Verification items for the finished model (mm, model axes). A direction names the side the tool comes from. Give positions to 0.01 mm unless a question says otherwise; leave off trailing zeros. Write each loop counter-clockwise with the first axis right and the second up, starting at its lowest first coordinate (ties: lowest second). Pieces come first, ordered by that corner, then holes. Notation, with made-up numbers: (4.5, 13.5) -> (9.5, 13.5) arc R19 cw to (9.5, 37.5) -> close; hole circle Ø5 at (36, 51.25). An arc over 180 degrees is marked (long way). Write item = value, one per line.
from build123d import *

# Parameters (mm, degrees)
PAD011_DEPTH                = 4.6
SKETCH016_W                 = 26.6
SKETCH016_H                 = 26.6
POCKET005_DEPTH             = 3.6
SKETCH018_R                 = 2.032
SKETCH018_R_2               = 0.832
PAD012_DEPTH                = 2
SKETCH018_MIRRORED013_2_R   = 2.032
SKETCH018_MIRRORED013_2_R_2 = 0.832
PAD012_MIRRORED013_2_DEPTH  = 2
SKETCH_R                    = 1.432
SKETCH_R_2                  = 0.832
PAD_DEPTH                   = 1.6
SKETCH_MIRRORED023_2_R      = 1.432
SKETCH_MIRRORED023_2_R_2    = 0.832
PAD_MIRRORED023_2_DEPTH     = 1.6
POCKET007_DEPTH             = 1.001
POCKET009_DEPTH             = 4
POCKET009_MIRRORED_2_DEPTH  = 4
FILLET014_R                 = 2


with BuildPart() as part:
    # Sketch015 → Pad011 (new body)
    with BuildSketch(Plane.XY):
        with BuildLine():
            Line((-13.3, 14.5), (13.3, 14.5))
            ThreePointArc((14.5, 13.3), (14.148528, 14.148528), (13.3, 14.5))
            Line((14.5, 13.3), (14.5, -13.3))
            ThreePointArc((13.3, -14.5), (14.148528, -14.148528), (14.5, -13.3))
            Line((13.3, -14.5), (-13.3, -14.5))
            ThreePointArc((-14.5, -13.3), (-14.148528, -14.148528), (-13.3, -14.5))
            Line((-14.5, -13.3), (-14.5, 13.3))
            ThreePointArc((-13.3, 14.5), (-14.148528, 14.148528), (-14.5, 13.3))
        make_face()
    extrude(amount=PAD011_DEPTH)

    # Sketch016 (on Face10 of Pad011) → Pocket005 (cut)
    with BuildSketch(Plane.XY.offset(4.6)):
        Rectangle(SKETCH016_W, SKETCH016_H)
    extrude(amount=-POCKET005_DEPTH, mode=Mode.SUBTRACT)

    # Sketch018 → Pad012 (join)
    with BuildSketch(Plane.XY.offset(1)):
        with Locations((10.16, 10.16)):
            Circle(SKETCH018_R)
        with Locations((10.16, 10.16)):
            Circle(SKETCH018_R_2, mode=Mode.SUBTRACT)
    pad012 = extrude(amount=PAD012_DEPTH)

    # Sketch018 Mirrored013 2 → Pad012 Mirrored013 2 (add)
    with BuildSketch(Plane(origin=(0, 0, 1), x_dir=(-1, 0, 0), z_dir=(0, 0, -1))):
        with Locations((10.16, 10.16)):
            Circle(SKETCH018_MIRRORED013_2_R)
        with Locations((10.16, 10.16)):
            Circle(SKETCH018_MIRRORED013_2_R_2, mode=Mode.SUBTRACT)
    pad012_mirrored013_2 = extrude(amount=-PAD012_MIRRORED013_2_DEPTH)

    # Mirrored014: Pad012, Pad012 Mirrored013 2 across Sketch018 H_Axis
    add(pad012.mirror(Plane(origin=(0, 0, 1), x_dir=(0, 0, 1), z_dir=(0, 1, 0))))
    add(pad012_mirrored013_2.mirror(Plane(origin=(0, 0, 1), x_dir=(0, 0, 1), z_dir=(0, 1, 0))))

    # Sketch (on Face22 of MultiTransform008) → Pad (join)
    with BuildSketch(Plane.XY.offset(3)):
        with Locations((10.16, 10.16)):
            Circle(SKETCH_R)
        with Locations((10.16, 10.16)):
            Circle(SKETCH_R_2, mode=Mode.SUBTRACT)
    pad = extrude(amount=PAD_DEPTH)

    # Sketch Mirrored023 2 → Pad Mirrored023 2 (add)
    with BuildSketch(Plane(origin=(0, 0, 3), x_dir=(-1, 0, 0), z_dir=(0, 0, -1))):
        with Locations((10.16, 10.16)):
            Circle(SKETCH_MIRRORED023_2_R)
        with Locations((10.16, 10.16)):
            Circle(SKETCH_MIRRORED023_2_R_2, mode=Mode.SUBTRACT)
    pad_mirrored023_2 = extrude(amount=-PAD_MIRRORED023_2_DEPTH)

    # Mirrored024: Pad, Pad Mirrored023 2 across Sketch H_Axis
    add(pad.mirror(Plane(origin=(0, 0, 3), x_dir=(0, 0, 1), z_dir=(0, 1, 0))))
    add(pad_mirrored023_2.mirror(Plane(origin=(0, 0, 3), x_dir=(0, 0, 1), z_dir=(0, 1, 0))))

    # Sketch020 (on Face15 of Pocket005) → Pocket007 (cut, through all)
    with BuildSketch(Plane.XY.offset(1)):
        with BuildLine():
            ThreePointArc((6.35, 6.35), (0, 12.7), (-6.35, 6.35))
            ThreePointArc((-6.35, 6.35), (-12.699991, 0), (-6.35, -6.35))
            ThreePointArc((-6.35, -6.35), (0, -12.7), (6.35, -6.35))
            ThreePointArc((6.35, -6.35), (12.7, 0), (6.35, 6.35))
        make_face()
    extrude(amount=-POCKET007_DEPTH, mode=Mode.SUBTRACT)

    # Sketch026 (on Face6 of Pocket007) → Pocket009 (cut)
    with BuildSketch(Plane.XZ.offset(14.5)):
        Polygon((14.5, 0), (13.799792, 1), (14.5, 2), align=None)
    pocket009 = extrude(amount=-POCKET009_DEPTH, mode=Mode.SUBTRACT)

    # Sketch026 Mirrored 2 → Pocket009 Mirrored 2 (cut)
    with BuildSketch(Plane(origin=(0, -14.5, 0), x_dir=(-1, 0, 0), z_dir=(0, 1, 0))):
        Polygon((14.5, 0), (13.799792, 1), (14.5, 2), align=None)
    pocket009_mirrored_2 = extrude(amount=POCKET009_MIRRORED_2_DEPTH, mode=Mode.SUBTRACT)

    # Mirrored022: Pocket009, Pocket009 Mirrored 2 across XZ
    add(pocket009.mirror(Plane.XZ), mode=Mode.SUBTRACT)
    add(pocket009_mirrored_2.mirror(Plane.XZ), mode=Mode.SUBTRACT)

    # Fillet014
    fillet014_edges = [part.edges().sort_by_distance(p)[0] for p in [
        (-6.35, 6.35, 0.5),
        (6.35, 6.35, 0.5),
        (-6.35, -6.35, 0.5),
        (6.35, -6.35, 0.5),
    ]]
    fillet(fillet014_edges, radius=FILLET014_R)


solid = part.part
Item 1: Go/stop test with flat-tipped pins: P1, Ø0.6, axis at x = -14, z = 1.5, coming from the -Y side; P2, Ø0.8, axis at x = 14, z = 1.5, coming from the -Y side; P3, Ø1.3, axis at x = -10.16, y = -10.16, coming from the +Z side. Record where each tip stops, or that it passes through.
Response values:
P1 = -14.43
P2 = -14.46
P3 = 1
Item 2: Sectioned sample at A-A on z = 3.55. Give the number of separate pieces and of enclosed holes in the cut face, then the cut area to 3 significant figures.
Response values:
separate_pieces = 5
enclosed_holes = 5
area = 149 mm^2
Item 3: Sectioned sample at B-B on x = 5.25. Record the cut outline in (y, z), then the cut area to 3 significant figures.
Response values:
outline = (-14.5, 0) -> (-9.92, 0) -> (-9.92, 1) -> (-13.3, 1) -> (-13.3, 4.6) -> (-14.5, 4.6) -> close; (9.92, 0) -> (14.5, 0) -> (14.5, 4.6) -> (13.3, 4.6) -> (13.3, 1) -> (9.92, 1) -> close
area = 17.8 mm^2
Item 4: Set-up check for faces 1 (the flat face through (14.145, 12.473, 1.493)), 2 (the flat face through (13.3, 0, 3)), 3 (the flat face through (-14.145, 12.473, 1.493)): record each of +Z, -Z, +X, -X, +Y, -Y from which the full face is reachable in a straight line by a thin tool's end or side.
Response values:
face_1 = +X, +Y
face_2 = +Z
face_3 = -X, +Y
Item 5: Material ranges on line 1 (Y direction, x = -10.16, z = 2.15); line 2 (Y direction, x = 10.16, z = 3.7), recorded low to high.
Response values:
line_1 = -14.5 to -13.3, -12.19 to -10.99, -9.33 to -8.13, 8.13 to 9.33, 10.99 to 12.19, 13.3 to 14.5
line_2 = -14.5 to -13.3, -11.59 to -10.99, -9.33 to -8.73, 8.73 to 9.33, 10.99 to 11.59, 13.3 to 14.5
Item 6: Mould release check, pull along Y, two halves, no side actions. Record for faces 4 (the flat face through (14.155, -12.473, 0.493)), 5 (the cylindrical face through (13.98, -14.29, 2.78)), 6 (the cylindrical face through (13.999, 14.275, 2.779)), 7 (the flat face through (0, -13.3, 3)): +Y half, -Y half, draft (parallel to the pull), parting line (faces both ways), or undercut.
Response values:
face_4 = draft
face_5 = -Y half
face_6 = +Y half
face_7 = undercut
